Read the model definition and answer for the solid it produces. Units are mm, in the model's axes. Give positions to 0.01 mm unless a question says otherwise; leave off trailing zeros. Order: outer loops, then holes, each group sorted by start corner. A loop starts at its lowest first (then second) coordinate and runs counter-clockwise, first axis right, second up. Notation, with made-up numbers: (23.5, 59.25) -> (47.5, 59.25) arc R22 ccw to (47.5, 71.25) -> close; hole circle Ø6 at (78.25, -30.75). An arc over 180 degrees is marked (long way). Answer as CSV lines item,"result". Start each with the question number.
1) Straight lines are drawn through the part: L1, parallel to Y at x = 0, z = 10; L2, parallel to Y at x = -13, z = -49; L3, parallel to X at y = 31, z = 29. For each, find the intervals that lie inside material, in ascending order. Write a range as from..to.
2) Flat-ended cylindrical pins translate along their axes: pin 1 Ø8 at (x, z) = (35.5, -49) entering from +Y; pin 2 Ø12 at (y, z) = (81.5, -59) entering from +X; pin 3 Ø2 at (x, z) = (55, 27) entering from +Y; pin 4 Ø10 at (y, z) = (31, 9.5) entering from -X. Find the tip coordinate at first contact, or state that the pin passes through.
3) The mould has two halves that part along Y. Classify faces 1 (the face through (-8.527, 92.126, -8.96)), 2 (the face through (15.804, 51.97, -116.907)), 3 (the face through (66.475, 48.115, -9.042)), 4 (the face through (51, 69, 53.946)): +Y half, -Y half, draft (parallel to the pull), parting line (faces both ways), or undercut.
4) Find section A-A (z = 15.5). Determine the outline of the cut face in (x, y), and give its area (3 significant figures).
```python
from build123d import *

# Parameters (mm, degrees)
REVOLVE_THIN3_OUTLINE_W   = 2.54
REVOLVE_THIN3_OUTLINE_H   = 76.976451611
REVOLVE_THIN3_OUTLINE_H_2 = 0.206366599
REVOLVE_THIN3_OUTLINE_H_3 = 0.02094686
SKETCH32_R                = 47.246273806
SKETCH32_R_2              = 1.041920848
BOSS_EXTRUDE1_DEPTH       = 2.54
FILLET1_R                 = 2.54
SKETCH33_W                = 85.158841119
SKETCH33_H                = 0.170915888
CUT_EXTRUDE1_DEPTH        = 108.458
FILLET2_R                 = 0.254
FILLET3_R                 = 0.254
SCALE3_SCALE              = 1.65
SKETCH35_W                = 53.780187303
SKETCH35_H                = 190.112658653
CUT_EXTRUDE2_DEPTH        = 201.422


# Read off the part's stored shape, not the designer's step: Revolve-Thin3
with BuildPart() as part:
    # Revolve-Thin3 outline → Revolve-Thin3 (revolve)
    with BuildSketch(Plane.XZ.offset(-16.473592108)):
        with Locations((40.968314643, -5.968874658)):
            Rectangle(REVOLVE_THIN3_OUTLINE_W, REVOLVE_THIN3_OUTLINE_H)
        with BuildLine():
            add(Edge.make_bspline(
                [(39.698314643, 32.519351147), (39.687726817, 32.588202211), (39.677799336, 32.656993484), (39.668523832, 32.725717746)],
                knots=[0, 0, 0, 0, 0.007277117, 0.007277117, 0.007277117, 0.007277117], degree=3))
            Line((39.698314643, 32.519351147), (39.698314643, 32.725717746))
            Line((39.698314643, 32.725717746), (39.668523832, 32.725717746))
        make_face()
        with Locations((40.968314643, 32.622534446)):
            Rectangle(REVOLVE_THIN3_OUTLINE_W, REVOLVE_THIN3_OUTLINE_H_2)
        with BuildLine():
            add(Edge.make_bspline(
                [(39.668523832, 32.725717746), (39.518472779, 33.837479263), (39.539043978, 34.931703978), (39.695973098, 35.985611225), (39.697140195, 35.99339708), (39.698314643, 36.001180261)],
                knots=[0.007277117, 0.007277117, 0.007277117, 0.007277117, 0.125, 0.125, 0.125876466, 0.125876466, 0.125876466, 0.125876466], degree=3))
            Line((39.668523832, 32.725717746), (39.698314643, 32.725717746))
            Line((39.698314643, 32.725717746), (39.698314643, 36.001180261))
        make_face()
        with BuildLine():
            Line((39.698314643, -44.478047324), (39.698314643, -44.457100464))
            add(Edge.make_bspline(
                [(39.697961573, -44.478047324), (39.698080508, -44.471066539), (39.698198198, -44.464084253), (39.698314643, -44.457100464)],
                knots=[0.999591782, 0.999591782, 0.999591782, 0.999591782, 1, 1, 1, 1], degree=3))
            Line((39.697961573, -44.478047324), (39.698314643, -44.478047324))
        make_face()
        with Locations((40.968314643, -44.467573894)):
            Rectangle(REVOLVE_THIN3_OUTLINE_W, REVOLVE_THIN3_OUTLINE_H_3)
        with BuildLine():
            Line((39.698314643, 36.001180261), (39.698314643, 32.725717746))
            Line((39.698314643, 32.725717746), (42.238314643, 32.725717746))
            add(Edge.make_bspline(
                [(42.238314643, 32.725717746), (42.054562539, 33.777592883), (42.068967464, 34.803136992), (42.238314643, 35.799403945)],
                knots=[0, 0, 0, 0, 0.141281123, 0.141281123, 0.141281123, 0.141281123], degree=3))
            Line((42.238314643, 35.799403945), (42.238314643, 42.203297665))
            add(Edge.make_bspline(
                [(39.698314643, 36.001180261), (39.864637797, 37.10341997), (40.178381679, 38.152034474), (41.000947274, 40.135916369), (41.510862605, 41.071843995), (42.130351801, 42.038577334), (42.184085036, 42.121152876), (42.238314643, 42.203297665)],
                knots=[0.125876466, 0.125876466, 0.125876466, 0.125876466, 0.25, 0.25, 0.375, 0.375, 0.386733849, 0.386733849, 0.386733849, 0.386733849], degree=3))
        make_face()
        with BuildLine():
            Line((39.698314643, -44.478047324), (39.697961573, -44.478047324))
            add(Edge.make_bspline(
                [(18.010435206, -70.677083721), (19.79573085, -70.522158772), (21.456515081, -70.25595625), (24.590707244, -69.498066317), (26.054293619, -68.998406284), (28.729976787, -67.78317439), (29.942341958, -67.068017905), (32.141805888, -65.420707287), (33.129574164, -64.488411909), (34.902639951, -62.386085615), (35.688102783, -61.215394241), (37.05999238, -58.60954034), (37.646016791, -57.174096931), (39.087083849, -52.452836699), (39.625242566, -48.746219412), (39.697961573, -44.478047324)],
                knots=[0.004627238, 0.004627238, 0.004627238, 0.004627238, 0.125, 0.125, 0.25, 0.25, 0.375, 0.375, 0.5, 0.5, 0.625, 0.625, 0.75, 0.75, 0.999591782, 0.999591782, 0.999591782, 0.999591782], degree=3))
            Line((18.010435206, -70.677083721), (18.010435206, -70.694456457))
            Line((18.010435206, -70.694456457), (28.462249201, -70.694456457))
            add(Edge.make_bspline(
                [(28.462249201, -70.694456457), (36.319875776, -67.117155429), (39.698314643, -58.770046926)],
                knots=[0.250450742, 0.250450742, 0.250450742, 0.688405646, 0.688405646, 0.688405646], degree=2))
            Line((39.698314643, -58.770046926), (39.698314643, -44.478047324))
        make_face()
        with BuildLine():
            Line((42.238314643, -44.478047324), (39.698314643, -44.478047324))
            Line((39.698314643, -44.478047324), (39.698314643, -58.770046926))
            add(Edge.make_bspline(
                [(39.698314643, -58.770046926), (42.101992439, -52.831280485), (42.238314643, -44.478047324)],
                knots=[0.688405646, 0.688405646, 0.688405646, 1, 1, 1], degree=2))
        make_face()
        with BuildLine():
            add(Edge.make_bspline(
                [(42.238314643, 42.203297665), (42.472937439, 42.558694673), (42.716851503, 42.906028704), (43.268191066, 43.654706519), (43.576088068, 44.050007388), (44.486136773, 45.194626874), (45.074219946, 45.904218472), (46.0952688, 47.247624232), (46.526137449, 47.880446647), (46.995778794, 48.764796386), (47.123505223, 49.048386117), (47.278542653, 49.476995244), (47.325447008, 49.628350247), (47.363757964, 49.77823029)],
                knots=[0.386733849, 0.386733849, 0.386733849, 0.386733849, 0.4375, 0.4375, 0.5, 0.5, 0.625, 0.625, 0.75, 0.75, 0.8125, 0.8125, 0.847702352, 0.847702352, 0.847702352, 0.847702352], degree=3))
            Line((42.238314643, 42.203297665), (42.238314643, 35.799403945))
            add(Edge.make_bspline(
                [(42.238314643, 35.799403945), (42.577155463, 37.792799485), (44.167905472, 40.904465888), (46.512712316, 43.628815223), (47.363757964, 44.722836867)],
                knots=[0.141281123, 0.141281123, 0.141281123, 0.141281123, 0.423965559, 0.610115154, 0.610115154, 0.610115154, 0.610115154], degree=3))
            Line((47.363757964, 44.722836867), (47.363757964, 49.77823029))
        make_face()
        with BuildLine():
            Line((18.010435206, -70.694456457), (18.010435206, -70.677083721))
            add(Edge.make_bspline(
                [(17.803998036, -70.694456457), (17.872994465, -70.688830195), (17.941806831, -70.683039176), (18.010435206, -70.677083721)],
                knots=[0, 0, 0, 0, 0.004627238, 0.004627238, 0.004627238, 0.004627238], degree=3))
            Line((17.803998036, -70.694456457), (18.010435206, -70.694456457))
        make_face()
        with BuildLine():
            add(Edge.make_bspline(
                [(47.363757964, 49.77823029), (47.393466178, 49.894454702), (47.418006992, 50.009792187), (47.482293388, 50.388738185), (47.501353806, 50.652055315), (47.481910982, 51.210629928), (47.44332582, 51.506604575), (47.363757964, 51.83451188)],
                knots=[0.847702352, 0.847702352, 0.847702352, 0.847702352, 0.875, 0.875, 0.9375, 0.9375, 1, 1, 1, 1], degree=3))
            Line((47.363757964, 49.77823029), (47.363757964, 44.722836867))
            add(Edge.make_bspline(
                [(47.363757964, 44.722836867), (48.462338755, 46.135065654), (49.427688757, 47.567830661), (49.832127601, 49.178979157)],
                knots=[0.610115154, 0.610115154, 0.610115154, 0.610115154, 0.850408223, 0.850408223, 0.850408223, 0.850408223], degree=3))
            Line((49.832127601, 49.178979157), (49.832127601, 51.83451188))
            Line((49.832127601, 51.83451188), (47.363757964, 51.83451188))
        make_face()
        Polygon((18.010435206, -70.694456457), (17.803998036, -70.694456457), (18.010435206, -73.226053521), align=None)
        with BuildLine():
            Line((28.462249201, -70.694456457), (18.010435206, -70.694456457))
            Line((18.010435206, -70.694456457), (18.010435206, -73.226053521))
            add(Edge.make_bspline(
                [(18.010435206, -73.226053521), (23.968753656, -72.740186943), (28.462249201, -70.694456457)],
                knots=[0, 0, 0, 0.250450742, 0.250450742, 0.250450742], degree=2))
        make_face()
        Polygon((49.832127601, 52.433470423), (47.363757964, 51.83451188), (49.832127601, 51.83451188), align=None)
        with BuildLine():
            Line((49.832127601, 51.83451188), (49.832127601, 49.178979157))
            add(Edge.make_bspline(
                [(49.832127601, 49.178979157), (49.962029278, 49.696463804), (50.0340657, 50.232351019), (50.034065718, 50.791871057)],
                knots=[0.850408223, 0.850408223, 0.850408223, 0.850408223, 0.927587932, 0.927587932, 0.927587932, 0.927587932], degree=3))
            add(Edge.make_bspline(
                [(50.034065718, 50.791871057), (50.034065729, 51.130381669), (50.007698462, 51.477542535), (49.951825757, 51.83451188)],
                knots=[0.927587932, 0.927587932, 0.927587932, 0.927587932, 0.974281793, 0.974281793, 0.974281793, 0.974281793], degree=3))
            Line((49.951825757, 51.83451188), (49.832127601, 51.83451188))
        make_face()
        with BuildLine():
            add(Edge.make_bspline(
                [(49.951825757, 51.83451188), (49.921051995, 52.031124695), (49.881327391, 52.230713035), (49.832127601, 52.433470423)],
                knots=[0.974281793, 0.974281793, 0.974281793, 0.974281793, 1, 1, 1, 1], degree=3))
            Line((49.832127601, 52.433470423), (49.832127601, 51.83451188))
            Line((49.832127601, 51.83451188), (49.951825757, 51.83451188))
        make_face()
    revolve(axis=Axis((0, 16.473592108, 0), (0, 0, 1)))

    # Sketch33 → Cut-Extrude1 (cut)
    with BuildSketch(Plane(origin=(0, 76.2, 0), x_dir=(1, 0, 0), z_dir=(0, 1, 0))):
        with Locations((-0.060456445, -32.78023641)):
            Rectangle(SKETCH33_W, SKETCH33_H)
    extrude(amount=-CUT_EXTRUDE1_DEPTH, mode=Mode.SUBTRACT)


with BuildPart() as body_2:
    # Sketch32 → Boss-Extrude1 (new body)
    with BuildSketch(Plane.XY.offset(52.433470423)):
        with Locations((0, 16.473592108)):
            Circle(SKETCH32_R)
        with Locations((0, 16.473592108)):
            Circle(SKETCH32_R_2, mode=Mode.SUBTRACT)
    extrude(amount=BOSS_EXTRUDE1_DEPTH)

    # Fillet1
    fillet1_edges = [body_2.edges().sort_by_distance(p)[0] for p in [
        (-47.246273806, 16.473592108, 54.973470423),
        (-1.041920848, 16.473592108, 54.973470423),
    ]]
    fillet(fillet1_edges, radius=FILLET1_R - 0.0001)  # a hair under: the kernel refuses the full size


with BuildPart() as cut_extrude1_piece_1:
    # of the separate pieces the step leaves, piece 1, a body of its own (cut_extrude1_pieces)
    add(part.part.solids().sort_by_distance((42.238314643, 16.473592108, 32.694778466))[0])

    # Fillet2
    fillet2_edges = [cut_extrude1_piece_1.edges().sort_by_distance(p)[0] for p in [
        (-42.238314643, 16.473592108, 32.694778466),
    ]]
    fillet(fillet2_edges, radius=FILLET2_R)


with BuildPart() as cut_extrude1_piece_2:
    # of the separate pieces the step leaves, piece 2, a body of its own (cut_extrude1_pieces)
    add(part.part.solids().sort_by_distance((42.215003382, 16.473592108, 32.865694354))[0])

    # Fillet3
    fillet3_edges = [cut_extrude1_piece_2.edges().sort_by_distance(p)[0] for p in [
        (-42.21500338, 16.473592107, 32.865694354),
    ]]
    fillet(fillet3_edges, radius=FILLET3_R)


with BuildPart() as body_2_1:
    # Scale3: scaled about (0, 0, 0)
    add(body_2.part.scale(SCALE3_SCALE))


with BuildPart() as cut_extrude1_piece_1_1:
    # Scale3: scaled about (0, 0, 0)
    add(cut_extrude1_piece_1.part.scale(SCALE3_SCALE))


with BuildPart() as cut_extrude1_piece_2_1:
    # Scale3: scaled about (0, 0, 0)
    add(cut_extrude1_piece_2.part.scale(SCALE3_SCALE))


with BuildPart() as cut_extrude2_tool:
    # Sketch35 → Cut-Extrude2 (new body)
    with BuildSketch(Plane(origin=(-101.6, 0, 0), x_dir=(0, 0, -1), z_dir=(1, 0, 0))):
        with Locations((-80.974469867, 30.532269515)):
            Rectangle(SKETCH35_W, SKETCH35_H)
    extrude(amount=CUT_EXTRUDE2_DEPTH)


with BuildPart() as body_2_2:
    add(body_2_1.part)

    # Cut-Extrude2: cut by cut_extrude2_tool
    add(cut_extrude2_tool.part, mode=Mode.SUBTRACT)


with BuildPart() as cut_extrude1_piece_2_2:
    add(cut_extrude1_piece_2_1.part)

    # Cut-Extrude2: cut by cut_extrude2_tool
    add(cut_extrude2_tool.part, mode=Mode.SUBTRACT)


solid = cut_extrude1_piece_1_1.part
```
Findings below:
1,L1,"-42.51..-38.32, 92.68..96.87"
1,L2,"-41.29..-37.02, 91.38..95.65"
1,L3,"-69.59..-65.39, 65.39..69.59"
2,pin 1,"y = 89.35"
2,pin 2,"x = 50.22"
2,pin 3,"y = 71.24"
2,pin 4,"x = -69.69"
3,face 1,"undercut"
3,face 2,"undercut"
3,face 3,"parting line"
3,face 4,"draft"
4,outline,"circle Ø139.39 at (0, 27.18); hole circle Ø131 at (0, 27.18)"
4,area,"1,780 mm²"
